```python
from build123d import *

# Parameters (mm, degrees)
CYLINDER005_R            = 1.6
CYLINDER005_DEPTH        = 30
PAD002_DEPTH             = 4
CLONE017_PLACEMENT_ANGLE = 60.399047773


with BuildPart() as finger_drill_master:
    # Cylinder005 → Cylinder005 (new body)
    with BuildSketch(Plane.XY.offset(-8)):
        Circle(CYLINDER005_R)
    extrude(amount=CYLINDER005_DEPTH)


with BuildPart() as clone006:
    # Clone006 base: copy of finger-drill-master
    add(finger_drill_master.part)


with BuildPart() as clone006_1:
    # Clone006 placement: moved
    add(clone006.part.moved(Location((40, 0, 0))))


with BuildPart() as fusion012:
    # Clone005 base: copy of finger-drill-master
    add(finger_drill_master.part)

    # Fusion012: union Clone006
    add(clone006_1.part)


with BuildPart() as clone_of_right_link:
    # Sketch002 → Pad002 (new body)
    with BuildSketch(Plane.XY):
        with BuildLine():
            ThreePointArc((0, 3.7), (-3.7, 0), (0, -3.7))
            Line((0, -3.7), (40, -3.7))
            ThreePointArc((40, -3.7), (43.7, 0), (40, 3.7))
            Line((0, 3.7), (40, 3.7))
        make_face()
    extrude(amount=PAD002_DEPTH)

    # Cut001: cut Fusion012
    add(fusion012.part, mode=Mode.SUBTRACT)


with BuildPart() as clone_of_right_link_1:
    # Clone017 placement: moved
    add(clone_of_right_link.part.moved(Location((216.2035278557, 248.9337248036, 4.3))).rotate(Axis((216.2035278557, 248.9337248036, 4.3), (0, 0, -1)), CLONE017_PLACEMENT_ANGLE))


with BuildPart() as clone_of_right_link_2:
    # Clone182 placement: moved
    add(clone_of_right_link_1.part.moved(Location((-14, -699, 7.3))))


solid = clone_of_right_link_2.part
```
Read the model definition and answer for the solid it produces. Units are mm, in the model's axes. Give positions to 0.01 mm unless a question says otherwise; leave off trailing zeros. Write each loop counter-clockwise with the first axis right and the second up, starting at its lowest first coordinate (ties: lowest second). Pieces come first, ordered by that corner, then holes. Notation, with made-up numbers: M 61,71.25 L 114,71.25 A27 ccw 114,106.25 Z; hole C -38,72.25 d7. An arc over 180 degrees is marked long. Put each result on its own line as item: value. Start each with the question number.
1. The part is cut by section C-C, the plane y = -463. Give the vertices of the cut face in (x, z), and give its area (3 significant figures).
2. The part is cut by section B-B, the plane x = 215.25. Give the vertices of the cut face in (y, z).
3. For a pull along Y with two mould halves and no side action, classify faces 1 (the cylindrical face through (223.72, -488.1, 13.57)), 2 (the flat face through (212, -467, 15.6)), 3 (the cylindrical face through (223.56, -484.93, 13.57)) as released by +Y, released by -Y, zero draft, split by the parting line, or undercut.
4. Each of these flat-tipped pins is pushed along its axis until it touches: pin 1 Ø2 at (x, z) = (217, 15) entering from +Y; pin 2 Ø1 at (y, z) = (-472, 13.5) entering from -X; pin 3 Ø1.5 at (y, z) = (-480.5, 15) entering from -X. Where does it stop, or does it pass through?
5. Consider line 1 along Y through (x, z) = (221.25, 11.8); line 2 along Y through (x, z) = (201.75, 12.65); line 3 along X through (y, z) = (-463.5, 14). Determine where each line is inside the solid, lowest interval first.
6. The part is cut by section A-A, the plane z = 12.75. Give the vertices of the cut face in (x, y).
Final values:
1. outline: M 205.3,11.6 L 213.81,11.6 L 213.81,15.6 L 205.3,15.6 Z
1. area: 34.0 mm²
2. outline: M -480.52,11.6 L -465.54,11.6 L -465.54,15.6 L -480.52,15.6 Z
3. face 1: split by the parting line
3. face 2: zero draft
3. face 3: undercut
4. pin 1: stops at y = -466.86
4. pin 2: stops at x = 210.12
4. pin 3: stops at x = 214.81
5. line 1: y = -488.48 to -486.28, -483.41 to -476.1
5. line 2: y = -456.76 to -451.6, -448.53 to -446.39
5. line 3: x = 205.58 to 214.09
6. outline: M 198.99,-451.89 L 218.74,-486.67 A3.7 ccw 225.18,-483.02 L 205.42,-448.24 A3.7 ccw Z; hole C 202.2,-450.07 d3.2; hole C 221.96,-484.85 d3.2
